```python
from build123d import *

# Parameters (mm, degrees)
ESQUISSE1_R             = 2.5
BOSS_EXTRU_1_DEPTH      = 20
ESQUISSE2_R             = 1.5
ENL_V_MAT_EXTRU_1_DEPTH = 10


with BuildPart() as part:
    # Esquisse1 → Boss.-Extru.1 (new body)
    with BuildSketch(Plane.XY):
        with BuildLine():
            ThreePointArc((-6, 0), (0, -6), (6, 0))
            Line((6, 0), (6, 2.5))
            Line((6, 2.5), (12, 2.5))
            Line((12, 2.5), (12, 12))
            Line((12, 12), (-12, 12))
            Line((-12, 12), (-12, 2.5))
            Line((-12, 2.5), (-6, 2.5))
            Line((-6, 2.5), (-6, 0))
        make_face()
        Circle(ESQUISSE1_R, mode=Mode.SUBTRACT)
    extrude(amount=-BOSS_EXTRU_1_DEPTH)

    # Esquisse2 → Enlèv. mat.-Extru.1 (cut)
    with BuildSketch(Plane.XZ.offset(-2.5)):
        with Locations(Location((-9, -10, 0), (0, 0, 270))):
            Circle(ESQUISSE2_R)
        with Locations(Location((9, -10, 0), (0, 0, 270))):
            Circle(ESQUISSE2_R)
    extrude(amount=-ENL_V_MAT_EXTRU_1_DEPTH, mode=Mode.SUBTRACT)


solid = part.part
```
Input: part model. Units: mm. Frame: model coordinates. A direction names the side the tool comes from. Coordinates: 2 decimals unless noted, no trailing zeros. Loops run counter-clockwise (first coordinate to the right, second up) from the corner with the lowest first, then second, coordinate; pieces in that order, holes last. Notation, with made-up numbers: (36, 1.25) - (65, 1.25) arc R24 cw to (65, 36.25) - close; hole circle Ø4 at (69, 50). An arc over 180 degrees is marked (long way). Answer in a Markdown table with one row per item.
(1) Cut plane C-C on z = -8. Output: boundary loops of the cut face in (x, y).
Model answer:
| item | result |
|---|---|
| outline | (-12, 2.5) - (-6, 2.5) - (-6, 0) arc R6 ccw to (6, 0) - (6, 2.5) - (12, 2.5) - (12, 12) - (-12, 12) - close; hole circle Ø5 at (0, 0) |
(2) Set-up query: faces 1 (the face through (6, 1, -10)), 2 (the face through (0, -6, -10)), 3 (the face through (-7, 2.5, -10)). Return all of +Z, -Z, +X, -X, +Y, -Y with unobstructed straight access to the full face (end or side cutting, diameter ignored); none if empty.
Model answer:
| item | result |
|---|---|
| face 1 | +Z, -Z, +X, -Y |
| face 2 | +Z, -Z, -Y |
| face 3 | +Z, -Z, -X, -Y |
(3) Material intervals for L1, parallel to X at y = 10, z = -10; L2, parallel to Y at x = 0, z = -13.25; L3, parallel to Y at x = -9.75, z = -14.75, sorted ascending. Write a range as from..to.
Model answer:
| item | result |
|---|---|
| L1 | x = -12..-10.5, -7.5..7.5, 10.5..12 |
| L2 | y = -6..-2.5, 2.5..12 |
| L3 | y = 2.5..12 |
(4) Cut plane D-D on y = 10.75. Output: boundary loops of the cut face in (x, z), plus the area to 3 significant figures.
Model answer:
| item | result |
|---|---|
| outline | (-12, -20) - (12, -20) - (12, 0) - (-12, 0) - close; hole circle Ø3 at (-9, -10); hole circle Ø3 at (9, -10) |
| area | 466 mm² |
(5) Mould query, pull axis Y, two halves, no side actions, for faces 4 (the face through (0, 12, -10)), 5 (the face through (11, 2.5, -10)), 6 (the face through (-0.54, -2.44, -9.86)), 7 (the face through (-12, 7, -10)). Classes: pulls with the +Y half, pulls with the -Y half, needs draft (parallel to the pull), parting line crosses it, or undercut.
Model answer:
| item | result |
|---|---|
| face 4 | pulls with the +Y half |
| face 5 | pulls with the -Y half |
| face 6 | undercut |
| face 7 | needs draft |
(6) Cut plane B-B on x = -9. Output: boundary loops of the cut face in (y, z).
Model answer:
| item | result |
|---|---|
| outline | (2.5, -20) - (12, -20) - (12, -11.5) - (2.5, -11.5) - close; (2.5, -8.5) - (12, -8.5) - (12, 0) - (2.5, 0) - close |
(7) Pin query (flat end, axial travel): P1, Ø1.5, axis at x = 4, z = -12.5, coming from the -Y side; P2, Ø6, axis at x = 6.5, z = -4.5, coming from the -Y side; P3, Ø5, axis at x = 9, z = -10, coming from the -Y side; P4, Ø4, axis at x = -9, z = -10, coming from the +Y side. Return the tip coordinate at first contact, or that it passes through.
Model answer:
| item | result |
|---|---|
| P1 | stops at y = -5.04 |
| P2 | stops at y = -4.87 |
| P3 | stops at y = 2.5 |
| P4 | stops at y = 12 |
(8) Cut plane A-A on z = -10. Output: boundary loops of the cut face in (x, y), plus the area to 3 significant figures.
Model answer:
| item | result |
|---|---|
| outline | (-12, 2.5) - (-10.5, 2.5) - (-10.5, 12) - (-12, 12) - close; (-7.5, 2.5) - (-6, 2.5) - (-6, 0) arc R6 ccw to (6, 0) - (6, 2.5) - (7.5, 2.5) - (7.5, 12) - (-7.5, 12) - close; (10.5, 2.5) - (12, 2.5) - (12, 12) - (10.5, 12) - close; hole circle Ø5 at (0, 0) |
| area | 238 mm² |
